from build123d import *

# Parameters (mm, degrees)
F0_W     = 38.1
F0_H     = 76.2
F1_DEPTH = 127
F2_R     = 25.4
F3_DEPTH = 101.6
F5_DEPTH = 76.2


with BuildPart() as f1:
    # F0 (on Front) → F1 (new body)
    with BuildSketch(Plane.XZ):
        with Locations((-90.780935, -13.071662)):
            Rectangle(F0_W, F0_H)
    extrude(amount=F1_DEPTH)

    # F2 (on face) → F3 (cut)
    with BuildSketch(Plane(origin=(-109.830935, 0, 0), x_dir=(0, -1, 0), z_dir=(-1, 0, 0))):
        with Locations((63.500002, -11.443584)):
            Circle(F2_R)
    extrude(amount=-F3_DEPTH, mode=Mode.SUBTRACT)

    # F4 (on face) → F5 (cut, through all)
    with BuildSketch(Plane.XY.offset(25.028338)):
        Polygon((-90.949364, -45.673328), (-102.886237, -52.387816), (-103.039757, -66.082696), (-91.256403, -73.063088), (-79.319529, -66.3486), (-79.16601, -52.65372), align=None)
    extrude(amount=-F5_DEPTH, mode=Mode.SUBTRACT)


solid = f1.part
Source: CAD feature listing. Evaluate the final solid. Frame: model axes, mm. A direction names the side the tool comes from. Coordinates: 2 decimals unless noted, no trailing zeros. Order: outer loops, then holes, each group sorted by start corner. A loop starts at its lowest first (then second) coordinate and runs counter-clockwise, first axis right, second up.
Item 1: Cut plane D-D (z = -40). Return loops of the section in (x, y), plus the area to 3 significant figures.
Output values:
outline: (-109.83, -127) - (-71.73, -127) - (-71.73, 0) - (-109.83, 0) - close; hole (-103.04, -66.08) - (-91.26, -73.06) - (-79.32, -66.35) - (-79.17, -52.65) - (-90.95, -45.67) - (-102.89, -52.39) - close
area: 4,350 mm2
Item 2: Cut plane A-A (z = -6.5). Return loops of the section in (x, y).
Output values:
outline: (-109.83, -127) - (-71.73, -127) - (-71.73, -88.41) - (-109.83, -88.41) - close; (-109.83, -38.59) - (-71.73, -38.59) - (-71.73, 0) - (-109.83, 0) - close
Item 3: Cut plane C-C (x = -81). Return loops of the section in (y, z), plus the area to 3 significant figures.
Output values:
outline: (-127, -51.17) - (-67.29, -51.17) - (-67.29, -36.56) arc R25.4 cw to (-67.29, 13.67) - (-67.29, 25.03) - (-127, 25.03) - close; (-51.57, -51.17) - (0, -51.17) - (0, 25.03) - (-51.57, 25.03) - (-51.57, 10.98) arc R25.4 cw to (-51.57, -33.87) - close
area: 7,230 mm2
Item 4: Cut plane B-B (y = -64). Return loops of the section in (x, z).
Output values:
outline: (-109.83, -51.17) - (-103.02, -51.17) - (-103.02, -36.84) - (-109.83, -36.84) - close; (-109.83, 13.95) - (-103.02, 13.95) - (-103.02, 25.03) - (-109.83, 25.03) - close; (-79.29, -51.17) - (-71.73, -51.17) - (-71.73, -36.84) - (-79.29, -36.84) - close; (-79.29, 13.95) - (-71.73, 13.95) - (-71.73, 25.03) - (-79.29, 25.03) - close
Item 5: Set-up query: faces 5 (the face through (-78, -63, 25.028)), 6 (the face through (-85.37, -69.75, -42.96)). Return all of +Z, -Z, +X, -X, +Y, -Y with unobstructed straight access to the full face (end or side cutting, diameter ignored); none if empty.
Output values:
face 5: +Z, +X, -X, +Y, -Y
face 6: +Z, -Z
Item 6: Material intervals for line 1 (Y direction, x = -100.5, z = -38.5); line 2 (Y direction, x = -74, z = 9); line 3 (Z direction, x = -105.5, y = -48), sorted ascending.
Output values:
line 1: y = -127 to -67.59, -51.05 to 0
line 2: y = -127 to -78.57, -48.43 to 0
line 3: z = -51.17 to -31.57, 8.68 to 25.03
Item 7: Pull-direction query (Y, two-part tool) for faces 1 (the face through (-109.831, -63, -39)), 2 (the face through (-91.048, -87.727, -3.814)), 3 (the face through (-85, -49.2, 18)), 4 (the face through (-91, 0, -13)); classes: pulls with the +Y half, pulls with the -Y half, needs draft (parallel to the pull), parting line crosses it, or undercut.
Output values:
face 1: needs draft
face 2: undercut
face 3: undercut
face 4: pulls with the +Y half
